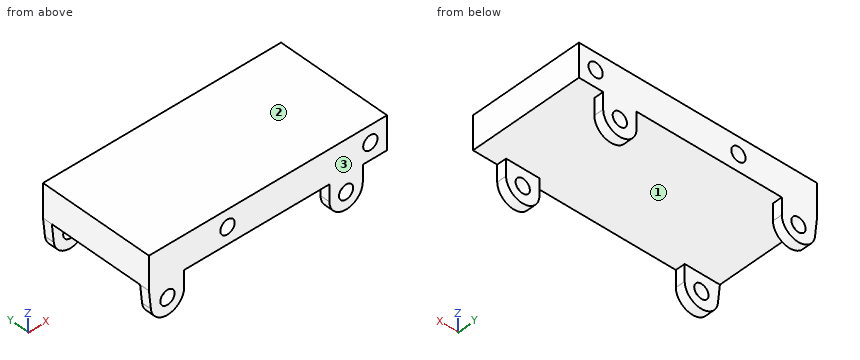
```python
from build123d import *

# Parameters (mm, degrees)
SKETCH2_W           = 50
SKETCH2_H           = 24
BOSS_EXTRUDE1_DEPTH = 7
SKETCH3_R           = 1.5
BOSS_EXTRUDE2_DEPTH = 2
BOSS_EXTRUDE3_START = -22
SKETCH3_2_R         = 1.5
BOSS_EXTRUDE3_DEPTH = 2
SKETCH5_R           = 1.5
CUT_EXTRUDE1_DEPTH  = 24
SKETCH6_R           = 1.5
CUT_EXTRUDE2_DEPTH  = 24


with BuildPart() as part:
    # Sketch2 → Boss-Extrude1 (new body)
    with BuildSketch(Plane.XY):
        with Locations((25, 12)):
            Rectangle(SKETCH2_W, SKETCH2_H)
    extrude(amount=BOSS_EXTRUDE1_DEPTH)

    # Sketch3 → Boss-Extrude2 (add)
    # profile 1 of 2: a face of its own
    with BuildSketch(Plane.XZ):
        with BuildLine():
            Line((7.39152842, -3.5), (7.39152842, 0))
            Line((7.39152842, 0), (0, 0))
            Line((0, 0), (0.411114128, -3.869751751))
            ThreePointArc((0.411114128, -3.869751751), (4.076663477, -6.995100143), (7.39152842, -3.5))
        make_face()
        with Locations(Location((3.89152842, -3.5, 0), (0, 0, 270))):
            Circle(SKETCH3_R, mode=Mode.SUBTRACT)
    # profile 2 of 2: a face of its own
    with BuildSketch(Plane.XZ):
        with BuildLine():
            Line((44.910130544, -3.5), (44.910130544, 0))
            Line((44.910130544, 0), (37.910130544, 0))
            Line((37.910130544, 0), (37.910130544, -3.5))
            ThreePointArc((37.910130544, -3.5), (41.410130544, -7), (44.910130544, -3.5))
        make_face()
        with Locations(Location((41.410130544, -3.5, 0), (0, 0, 270))):
            Circle(SKETCH3_R, mode=Mode.SUBTRACT)
    extrude(amount=-BOSS_EXTRUDE2_DEPTH)

    # Sketch3<2> → Boss-Extrude3 (add)
    # profile 1 of 2: a face of its own
    with BuildSketch(Plane.XZ.offset(BOSS_EXTRUDE3_START)):
        with BuildLine():
            Line((7.39152842, -3.5), (7.39152842, 0))
            Line((7.39152842, 0), (0, 0))
            Line((0, 0), (0.411114128, -3.869751751))
            ThreePointArc((0.411114128, -3.869751751), (4.076663477, -6.995100143), (7.39152842, -3.5))
        make_face()
        with Locations(Location((3.89152842, -3.5, 0), (0, 0, 270))):
            Circle(SKETCH3_2_R, mode=Mode.SUBTRACT)
    # profile 2 of 2: a face of its own
    with BuildSketch(Plane.XZ.offset(BOSS_EXTRUDE3_START)):
        with BuildLine():
            Line((44.910130544, -3.5), (44.910130544, 0))
            Line((44.910130544, 0), (37.910130544, 0))
            Line((37.910130544, 0), (37.910130544, -3.5))
            ThreePointArc((37.910130544, -3.5), (41.410130544, -7), (44.910130544, -3.5))
        make_face()
        with Locations(Location((41.410130544, -3.5, 0), (0, 0, 270))):
            Circle(SKETCH3_2_R, mode=Mode.SUBTRACT)
    extrude(amount=-BOSS_EXTRUDE3_DEPTH)

    # Sketch5 → Cut-Extrude1 (cut)
    with BuildSketch(Plane.XZ):
        with Locations(Location((46.5, 3.5, 0), (0, 0, 270))):
            Circle(SKETCH5_R)
    extrude(amount=-CUT_EXTRUDE1_DEPTH, mode=Mode.SUBTRACT)

    # Sketch6 → Cut-Extrude2 (cut)
    with BuildSketch(Plane.XZ):
        with Locations(Location((16.5, 3.5, 0), (0, 0, 270))):
            Circle(SKETCH6_R)
    extrude(amount=-CUT_EXTRUDE2_DEPTH, mode=Mode.SUBTRACT)


solid = part.part
```
Geometry: final body of the model. Coordinates: model frame, mm. Face numbers are marked on the shaded views. Round coordinates to 2 decimals unless told otherwise and drop trailing zeros. Write each loop counter-clockwise with the first axis right and the second up, starting at its lowest first coordinate (ties: lowest second). Pieces come first, ordered by that corner, then holes.
Item 1: Section query A-A (x = 16.5). Return loops of the section in (y, z).
Item 2: Pin query (flat end, axial travel): P1, Ø1.6, axis at y = 23, z = -1.5, coming from the +X side; P2, Ø8, axis at x = 30, y = 18.5, coming from the -Z side. Return the tip coordinate at first contact, or that it passes through.
Item 3: Section query D-D (y = 22.5). Return loops of the section in (x, z), plus the area to 3 significant figures.
Item 4: Material intervals for L1, parallel to X at y = 13.25, z = 3.5; L2, parallel to Y at x = 5, z = -1.5; L3, parallel to X at y = 0.7, z = -3.5, sorted ascending.
Item 5: Mould query, pull axis Y, two halves, no side actions, for the marked faces 1, 2 and 3. Classes: +Y half, -Y half, draft (parallel to the pull), parting line (faces both ways), or undercut.
Item 6: Section query C-C (y = 10.25). Return loops of the section in (x, z).
Item 7: Section query B-B (z = 3.5). Return loops of the section in (x, y).
Completed:
1. outline: (0, 0) - (24, 0) - (24, 2) - (0, 2) - close; (0, 5) - (24, 5) - (24, 7) - (0, 7) - close
2. P1: stops at x = 44.91
2. P2: stops at z = 0
3. outline: (0, 0) - (0.41, -3.87) arc R3.5 ccw to (7.39, -3.5) - (7.39, 0) - (37.91, 0) - (37.91, -3.5) arc R3.5 ccw to (44.91, -3.5) - (44.91, 0) - (50, 0) - (50, 7) - (0, 7) - close; hole circle Ø3 at (3.89, -3.5); hole circle Ø3 at (16.5, 3.5); hole circle Ø3 at (41.41, -3.5); hole circle Ø3 at (46.5, 3.5)
3. area: 410 mm2
4. L1: x = 0 to 15, 18 to 45, 48 to 50
4. L2: y = 0 to 2, 22 to 24
4. L3: x = 0.37 to 2.39, 5.39 to 7.39, 37.91 to 39.91, 42.91 to 44.91
5. face 1: undercut
5. face 2: draft
5. face 3: -Y half
6. outline: (0, 0) - (50, 0) - (50, 7) - (0, 7) - close; hole circle Ø3 at (16.5, 3.5); hole circle Ø3 at (46.5, 3.5)
7. outline: (0, 0) - (15, 0) - (15, 24) - (0, 24) - close; (18, 0) - (45, 0) - (45, 24) - (18, 24) - close; (48, 0) - (50, 0) - (50, 24) - (48, 24) - close
